The model under review builds one solid part; all positions refer to its coordinate system, in mm. A direction names the side the tool comes from. Give positions to 0.01 mm unless a question says otherwise; leave off trailing zeros. Order: outer loops, then holes, each group sorted by start corner. A loop starts at its lowest first (then second) coordinate and runs counter-clockwise, first axis right, second up. Notation, with made-up numbers: (-7, 23) - (47, 23) arc R33 cw to (47, 52) - close; hole circle Ø2 at (4.25, -15.5). An arc over 180 degrees is marked (long way). Put each result on its own line as item: value.
```python
from build123d import *

# Parameters (mm, degrees)
SKETCH001_R     = 7.5
PAD_DEPTH       = 50
POCKET_DEPTH    = 93.668
SKETCH002_R     = 3.125
POCKET001_DEPTH = 61.197951
SKETCH003_R     = 1.7
POCKET002_DEPTH = 61.197951
SKETCH004_R     = 2.625
POCKET003_DEPTH = 4
POCKET004_DEPTH = 2.65
SKETCH006_W     = 90
SKETCH006_H     = 15
POCKET005_DEPTH = 5


with BuildPart() as part:
    # Sketch001 → Pad (new body)
    with BuildSketch(Plane.XZ.offset(-9.25)):
        with BuildLine():
            Line((168.894231, 39), (211.105769, 39))
            Line((212, 36), (211.105769, 39))
            Line((212, 36), (236.667, 36))
            Line((235, 39), (236.667, 36))
            Line((233, 41), (235, 39))
            Line((217, 41), (233, 41))
            Line((213.125, 54), (217, 41))
            Line((201.125, 54), (213.125, 54))
            ThreePointArc((201.125, 54), (190, 61.196951), (178.875, 54))
            Line((166.875, 54), (178.875, 54))
            Line((166.875, 54), (163, 41))
            Line((163, 41), (147, 41))
            Line((145, 39), (147, 41))
            Line((145, 39), (143.333, 36))
            Line((143.333, 36), (168, 36))
            Line((168.894231, 39), (168, 36))
        make_face()
        with Locations((190, 49)):
            Circle(SKETCH001_R, mode=Mode.SUBTRACT)
    extrude(amount=PAD_DEPTH)

    # Sketch → Pocket (cut, through all)
    with BuildSketch(Plane.YZ.offset(143)):
        Polygon((4.25, 36), (9.25, 39), (9.25, 36), align=None)
        Polygon((-35.6, 36), (-40.75, 39), (-40.75, 36), align=None)
    extrude(amount=POCKET_DEPTH, mode=Mode.SUBTRACT)

    # Sketch002 → Pocket001 (cut, through all)
    with BuildSketch(Plane.XY):
        with Locations((155, -7)):
            Circle(SKETCH002_R)
        with Locations((155, -25)):
            Circle(SKETCH002_R)
        with Locations((225, -7)):
            Circle(SKETCH002_R)
        with Locations((225, -25)):
            Circle(SKETCH002_R)
    extrude(amount=POCKET001_DEPTH, mode=Mode.SUBTRACT)

    # Sketch003 → Pocket002 (cut, through all)
    with BuildSketch(Plane.XY):
        with Locations((173, 2)):
            Circle(SKETCH003_R)
        with Locations((173, -16)):
            Circle(SKETCH003_R)
        with Locations((173, -34)):
            Circle(SKETCH003_R)
        with Locations((207, 2)):
            Circle(SKETCH003_R)
        with Locations((207, -16)):
            Circle(SKETCH003_R)
        with Locations((207, -34)):
            Circle(SKETCH003_R)
    extrude(amount=POCKET002_DEPTH, mode=Mode.SUBTRACT)

    # Sketch004 → Pocket003 (cut)
    with BuildSketch(Plane.XY.offset(54)):
        with Locations((173, 2)):
            Circle(SKETCH004_R)
        with Locations((207, -16)):
            Circle(SKETCH004_R)
        with Locations((173, -16)):
            Circle(SKETCH004_R)
        with Locations((173, -34)):
            Circle(SKETCH004_R)
        with Locations((207, -34)):
            Circle(SKETCH004_R)
        with Locations((207, 2)):
            Circle(SKETCH004_R)
    extrude(amount=-POCKET003_DEPTH, mode=Mode.SUBTRACT)

    # Sketch005 → Pocket004 (cut)
    with BuildSketch(Plane.XY.offset(41)):
        Polygon((174.7, 4.944486), (171.3, 4.944486), (162.8, 4.944486), (162.8, -0.944486), (171.3, -0.944486), (174.7, -0.944486), (176.4, 2), align=None)
        Polygon((176.4, -16), (174.7, -13.055514), (171.3, -13.055514), (162.8, -13.055514), (162.8, -18.944486), (171.3, -18.944486), (174.7, -18.944486), align=None)
        Polygon((176.4, -34), (174.7, -31.055514), (171.3, -31.055514), (162.8, -31.055514), (162.8, -36.944486), (171.3, -36.944486), (174.7, -36.944486), align=None)
        Polygon((203.6, 2), (205.3, -0.944486), (208.7, -0.944486), (217.2, -0.944486), (217.2, 4.944486), (208.7, 4.944486), (205.3, 4.944486), align=None)
        Polygon((203.6, -16), (205.3, -18.944486), (208.7, -18.944486), (217.2, -18.944486), (217.2, -13.055514), (208.7, -13.055514), (205.3, -13.055514), align=None)
        Polygon((203.6, -34), (205.3, -36.944486), (208.7, -36.944486), (217.2, -36.944486), (217.2, -31.055514), (208.7, -31.055514), (205.3, -31.055514), align=None)
    extrude(amount=POCKET004_DEPTH, mode=Mode.SUBTRACT)

    # Sketch006 → Pocket005 (cut)
    with BuildSketch(Plane.XZ.offset(-26.5)):
        with Locations((190, 54.5)):
            Rectangle(SKETCH006_W, SKETCH006_H)
    extrude(amount=POCKET005_DEPTH, mode=Mode.SUBTRACT)


solid = part.part
```
(1) Take a section at D-D, the plane z = 58. Write out the cut boundary in (x, y).
The answers:
outline: (181.77, -40.75) - (198.23, -40.75) - (198.23, 9.25) - (181.77, 9.25) - close
(2) The part is to be moulded in two halves that separate along X. For faces 6 (the flat face through (204.438, -17.452, 42.306)), 7 (the flat face through (170, -15, 54)), 8 (the cylindrical face through (196.93, -15.4, 46.13)), say which applies: pulls with the +X half, pulls with the -X half, needs draft (parallel to the pull), parting line crosses it, or undercut.
The answers:
face 6: pulls with the +X half
face 7: needs draft
face 8: undercut
(3) For faces 1 (the flat face through (221, -15, 41)), 2 (the flat face through (209, -16, 50)), 3 (the flat face through (175.562, -32.548, 42.306)), 4 (the flat face through (189, -40.75, 40)), 5 (the cylindrical face through (174.62, -15.49, 46.78)), list the 3-axis set-ups (+Z, -Z, +X, -X, +Y, -Y) from which the entire face can be reached by the end or side of a thin tool; tool diameter is ignored.
The answers:
face 1: +X
face 2: +Z
face 3: -X
face 4: +Z, -Z, +X, -X, -Y
face 5: +Z, -Z
(4) Wall thickness on L1, parallel to Y at x = 173, z = 48; L2, parallel to X at y = -25, z = 38.4 (3 decimals); L3, parallel to X at y = -34, z = 39.4: over which ranges is each line inside the solid? List them lowest first.
The answers:
L1: -40.75 to -35.7, -32.3 to -17.7, -14.3 to 0.3, 3.7 to 9.25
L2: 144.667 to 151.875, 158.125 to 168.715, 211.285 to 221.875, 228.125 to 235.333
L3: 145.4 to 171.3, 174.7 to 205.3, 208.7 to 234.6
(5) Take a section at C-C, the plane y = -2. Write out the cut boundary in (x, z) (3 decimals), then the cut area to 3 significant figures.
The answers:
outline: (143.333, 36) - (168, 36) - (168.894, 39) - (211.106, 39) - (212, 36) - (236.667, 36) - (235, 39) - (233, 41) - (217, 41) - (213.125, 54) - (201.125, 54) arc R12.197 ccw to (178.875, 54) - (166.875, 54) - (163, 41) - (147, 41) - (145, 39) - close; hole circle Ø15 at (190, 49)
area: 912 mm^2
(6) Take a section at A-A, the plane y = -7. Write out the cut boundary in (x, z) (3 decimals).
The answers:
outline: (143.333, 36) - (151.875, 36) - (151.875, 41) - (147, 41) - (145, 39) - close; (158.125, 36) - (168, 36) - (168.894, 39) - (211.106, 39) - (212, 36) - (221.875, 36) - (221.875, 41) - (217, 41) - (213.125, 54) - (201.125, 54) arc R12.197 ccw to (178.875, 54) - (166.875, 54) - (163, 41) - (158.125, 41) - close; (228.125, 36) - (236.667, 36) - (235, 39) - (233, 41) - (228.125, 41) - close; hole circle Ø15 at (190, 49)
(7) Take a section at B-B, the plane x = 225. Write out the cut boundary in (y, z) (3 decimals).
The answers:
outline: (-40.75, 39) - (-35.6, 36) - (-28.125, 36) - (-28.125, 41) - (-40.75, 41) - close; (-21.875, 36) - (-10.125, 36) - (-10.125, 41) - (-21.875, 41) - close; (-3.875, 36) - (4.25, 36) - (9.25, 39) - (9.25, 41) - (-3.875, 41) - close
(8) Clearance check with flat-ended pins moving along their axes: pin 1 Ø10 at (x, y) = (193, -15.5) entering from +Z; pin 2 Ø1 at (x, y) = (154, -18) entering from +Z; pin 3 Ø6 at (x, y) = (207, -16) entering from -Z; pin 4 Ø2 at (y, z) = (-6.5, 55.5) entering from +X. State where each tip first meets the part, or that it passes through.
The answers:
pin 1: z = 61.2
pin 2: z = 41
pin 3: z = 39
pin 4: x = 200.89
